Could you check a few things on this model? Use its own coordinates, in mm. A direction names the side the tool comes from. Coordinates: 2 decimals unless noted, no trailing zeros. Write each loop counter-clockwise with the first axis right and the second up, starting at its lowest first coordinate (ties: lowest second). Pieces come first, ordered by that corner, then holes.
Item 1: I want a section at C-C on z = 9. Please give me the cut outline in (x, y).
Item 2: I want a section at B-B on y = -15.5. Please give me the cut outline in (x, z), then the cut area to 3 significant figures.
Item 3: For P1, Ø9.5, axis at x = 4, z = 10, coming from the -Y side, with a flat end and sliding along its axis, tell me the tip position at first contact or that it passes through.
Item 4: I want a section at D-D on x = -5.5. Please give me the cut outline in (y, z).
Item 5: Which directions (+Z, -Z, +X, -X, +Y, -Y) give clear straight access to the entire face, cutting with the end or side of a thin tool? Please do faces 1 (the cylindrical face through (22.627, 0.049, 4.607)), 2 (the flat face through (0, -2.5, 10)), 3 (the flat face through (0, 2.5, 10)).
Item 6: If I drill on probe 1 along Z at (x, y) = (15, 20.5); probe 2 along Y at (x, z) = (19, 4.75); probe 3 along X at (y, z) = (-0.5, 7.75), over which ranges is the centre line in solid material (lowest first)?
Item 7: I want a section at A-A on x = 24.5. Please give me the cut outline in (y, z).
from build123d import *

# Parameters (mm, degrees)
AUFSATZ_LINEAR_AUSTRAGEN1_DEPTH = 2
SKIZZE2_W                       = 25
SKIZZE2_H                       = 5
AUFSATZ_LINEAR_AUSTRAGEN2_DEPTH = 20
VERRUNDUNG1_R                   = 20
VERRUNDUNG2_R                   = 1
VERRUNDUNG3_R                   = 20
VERRUNDUNG4_R                   = 10


# Some blends are built 0.0001 mm under size
with BuildPart() as part:
    # Skizze1 → Aufsatz-Linear austragen1 (new body)
    with BuildSketch(Plane.XY):
        with BuildLine():
            Line((-32.5, -33.5), (32.5, -33.5))
            ThreePointArc((32.5, -33.5), (33.207106781, -33.207106781), (33.5, -32.5))
            Line((33.5, -32.5), (33.5, 32.5))
            ThreePointArc((33.5, 32.5), (33.207106781, 33.207106781), (32.5, 33.5))
            Line((32.5, 33.5), (-32.5, 33.5))
            ThreePointArc((-32.5, 33.5), (-33.207106781, 33.207106781), (-33.5, 32.5))
            Line((-33.5, 32.5), (-33.5, -32.5))
            ThreePointArc((-33.5, -32.5), (-33.207106781, -33.207106781), (-32.5, -33.5))
        make_face()
    extrude(amount=AUFSATZ_LINEAR_AUSTRAGEN1_DEPTH)

    # Skizze2 → Aufsatz-Linear austragen2 (add)
    with BuildSketch(Plane.XY.offset(2)):
        Rectangle(SKIZZE2_W, SKIZZE2_H)
    extrude(amount=AUFSATZ_LINEAR_AUSTRAGEN2_DEPTH)

    # Verrundung1
    verrundung1_edges = [part.edges().sort_by_distance(p)[0] for p in [
        (-12.5, 0, 2),
        (12.5, 0, 2),
    ]]
    fillet(verrundung1_edges, radius=VERRUNDUNG1_R - 0.0001)  # a hair under: the kernel refuses the full size

    # Verrundung2
    verrundung2_edges = [part.edges().sort_by_distance(p)[0] for p in [
        (0, 2.5, 2),
        (0, -2.5, 2),
    ]]
    fillet(verrundung2_edges, radius=VERRUNDUNG2_R)

    # Verrundung3
    # the kernel refuses this fillet: 20 mm, written as the material it takes off along each edge
    with BuildSketch(Plane(origin=(-12.5, 39.102646041, 22), x_dir=(1, 0, 0), z_dir=(0, -1, 0)), Plane(origin=(12.5, -39.102646041, 22), x_dir=(-1, 0, 0), z_dir=(0, 1, 0))) as verrundung3_piece_1:
        with BuildLine():
            CenterArc((14.641058416, -20), VERRUNDUNG3_R, 90, 60.0000827)
            Line((-2.679464093, -10.000025), (-4.411516344, -9.0000275))
            ThreePointArc((-4.411516344, -9.0000275), (-2, -0.0001), (-2, 0))
            Line((-2, 0), (0, 2))
            Line((0, 2), (14.641058416, 2))
            Line((14.641058416, 2), (14.641058416, 0))
        make_face()
    extrude(amount=78.205292082, mode=Mode.SUBTRACT)

    # Verrundung4
    verrundung4_edges = [part.edges().sort_by_distance(p)[0] for p in [
        (0, 0, 21.885066479),
    ]]
    fillet(verrundung4_edges, radius=VERRUNDUNG4_R)


solid = part.part
Response values:
1. outline: (-17.3, -2.5) - (17.3, -2.5) - (17.3, 2.5) - (-17.3, 2.5) - close
2. outline: (-33.5, 0) - (33.5, 0) - (33.5, 2) - (-33.5, 2) - close
2. area: 134 mm2
3. P1: stops at y = -2.5
4. outline: (-33.5, 0) - (33.5, 0) - (33.5, 2) - (3.5, 2) arc R1 cw to (2.5, 3) - (2.5, 20.48) - (-2.5, 20.48) - (-2.5, 3) arc R1 cw to (-3.5, 2) - (-33.5, 2) - close
5. face 1: +Z, +X, +Y, -Y
5. face 2: +Z, +X, -X, -Y
5. face 3: +Z, +X, -X, +Y
6. probe 1: z = 0 to 2
6. probe 2: y = -2.5 to 2.5
6. probe 3: x = -18.47 to 18.47
7. outline: (-33.5, 0) - (33.5, 0) - (33.5, 2) - (3.5, 2) arc R1 cw to (2.5, 3) - (2.5, 3.67) - (-2.5, 3.67) - (-2.5, 3) arc R1 cw to (-3.5, 2) - (-33.5, 2) - close
